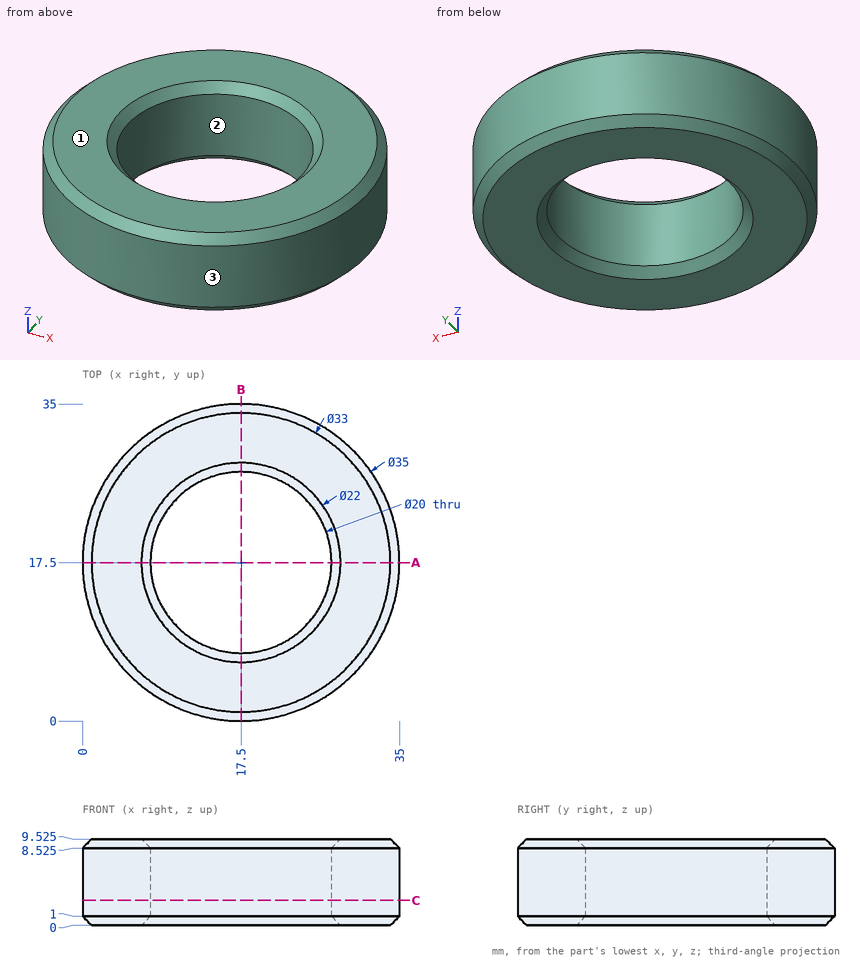
Study the drawing (mm; zero at the part's minimum x, y, z) and answer. Give positions to 0.01 mm unless a question says otherwise; leave off trailing zeros. Write each loop counter-clockwise with the first axis right and the second up, starting at its lowest first coordinate (ties: lowest second). Pieces come first, ordered by that corner, then holes.
(1) Straight lines are drawn through the part: line 1 (Y direction, x = 17.5, z = 6); line 2 (X direction, y = 11, z = 8.25); line 3 (X direction, y = 14.5, z = 4.5). For each, find the intervals that lie inside material, in ascending order.
Final values:
line 1: y = 0 to 7.5, 27.5 to 35
line 2: x = 1.25 to 9.9, 25.1 to 33.75
line 3: x = 0.26 to 7.96, 27.04 to 34.74
(2) The part is cut by section A-A on y = 17.5. Write down the section's boundary in (x, z) (3 decimals), plus the area to 3 significant figures.
Final values:
outline: (0, 1) - (1, 0) - (6.5, 0) - (7.5, 1) - (7.5, 8.525) - (6.5, 9.525) - (1, 9.525) - (0, 8.525) - close; (27.5, 1) - (28.5, 0) - (34, 0) - (35, 1) - (35, 8.525) - (34, 9.525) - (28.5, 9.525) - (27.5, 8.525) - close
area: 139 mm2
(3) The part is cut by section C-C on z = 2.75. Write down the section's boundary in (x, y).
Final values:
outline: circle Ø35 at (17.5, 17.5); hole circle Ø20 at (17.5, 17.5)
(4) Flat-ended cylindrical pins translate along their axes: pin 1 Ø2 at (x, z) = (21.5, 6.5) entering from -Y; pin 2 Ø4 at (x, z) = (13, 8) entering from +Y; pin 3 Ø2 at (x, z) = (14, 8.5) entering from -Y; pin 4 Ø2 at (x, y) = (22.5, 8) entering from +Z (3 decimals). Find the tip coordinate at first contact, or state that the pin passes through.
Final values:
pin 1: stops at y = 0.26
pin 2: stops at y = 34.82
pin 3: stops at y = 0.18
pin 4: stops at z = 9.525
(5) The mould has two halves that part along Y. Classify the marked faces 1, 2 and 3: pulls with the +Y half, pulls with the -Y half, needs draft (parallel to the pull), parting line crosses it, or undercut.
Final values:
face 1: needs draft
face 2: undercut
face 3: parting line crosses it
